from build123d import *

# Parameters (mm, degrees)
F2_DEPTH = 1.3
F4_DEPTH = 1.7
F6_DEPTH = 12.5


# Not quite as in the source:
# - a feature of the source that left no trace in its solid (it failed there, or was rolled back) is left out


with BuildPart() as f2:
    # F1 (on Top) → F2 (new body)
    with BuildSketch(Plane.XY):
        with BuildLine():
            Line((-5.1537473182, 3.6727124144), (-5.7416372565, -3.0469003289))
            ThreePointArc((-5.7416372565, -3.0469003289), (0, -6.5), (5.7416372565, -3.0469003289))
            Line((5.7416372565, -3.0469003289), (5.1537473182, 3.6727124144))
            Line((5.1537473182, 3.6727124144), (3.4859795486, 4.7765922388))
            Line((3.4859795486, 4.7765922388), (2.7272692442, 2.9260899627))
            ThreePointArc((2.7272692442, 2.9260899627), (0, -4), (-2.7272692442, 2.9260899627))
            Line((-2.7272692442, 2.9260899627), (-3.4859795486, 4.7765922388))
            Line((-3.4859795486, 4.7765922388), (-5.1537473182, 3.6727124144))
        make_face()
    extrude(amount=F2_DEPTH)

    # F3 (on face) → F4 (join)
    with BuildSketch(Plane.XY.offset(1.3)):
        with BuildLine():
            Line((-4.6721311475, -3.2651478589), (-5.3278688525, -3.723414225))
            ThreePointArc((-5.3278688525, -3.723414225), (0, -6.5), (5.3278688525, -3.723414225))
            Line((5.3278688525, -3.723414225), (4.6721311475, -3.2651478589))
            ThreePointArc((4.6721311475, -3.2651478589), (0, -5.7), (-4.6721311475, -3.2651478589))
        make_face()
    extrude(amount=F4_DEPTH)

    # F5 (on Right) → F6 (cut, symmetric)
    with BuildSketch(Plane.YZ):
        Polygon((6.7765922388, 1.3), (2.9260899627, 1.3), (6.7765922388, -0.9230885256), align=None)
    extrude(amount=F6_DEPTH, both=True, mode=Mode.SUBTRACT)


solid = f2.part
Geometry check sheet. Reference: the model listing, model coordinates, mm. A direction names the side the tool comes from. Round coordinates to 2 decimals unless told otherwise and drop trailing zeros. Loops run counter-clockwise (first coordinate to the right, second up) from the corner with the lowest first, then second, coordinate; pieces in that order, holes last.
Item 1: Access from +Z, -Z, +X, -X, +Y, -Y to the whole of each face (thin tool, end or side, straight path). Record for faces 1 (the flat face through (-0.1, -4.2, 1.3)), 2 (the flat face through (0, -6, 3)), 3 (the flat face through (3.03, 3.66, 0.5)).
Item 2: Cross-section at A-A on x = 0. Record the boundary of the cut face in (y, z), then the cut area to 3 significant figures.
Item 3: Gauge pin test, flat ends, axial feed: pin 1 (6.5 mm diameter, centred on x = 0, y = 0, fed in from +Z); pin 2 (3 mm diameter, centred on x = -2.5, y = -0.5, fed in from +Z); pin 3 (1.5 mm diameter, centred on x = 0.5, z = 1.5, fed in from +Y). Record the tip position at first contact, or that the pin passes through.
Item 4: Cross-section at C-C on z = 1.1. Record the boundary of the cut face in (x, y).
Item 5: Cross-section at D-D on x = 1.5. Record the boundary of the cut face in (y, z), then the cut area to 3 significant figures.
Item 6: Cross-section at B-B on y = 0. Record the boundary of the cut face in (x, z).
Item 7: Thickness scan on line 1 (Y direction, x = 0, z = 1.05); line 2 (Z direction, x = 3, y = -4.5); line 3 (X direction, y = 0, z = 0.5). Record the ranges inside material, lowest first.
Answer sheet:
1. face 1: +Z, +Y
1. face 2: +Z, +X, -X, +Y, -Y
1. face 3: +Z, -Z, +Y
2. outline: (-6.5, 0) - (-4, 0) - (-4, 1.3) - (-5.7, 1.3) - (-5.7, 3) - (-6.5, 3) - close
2. area: 4.61 mm2
3. pin 1: passes through
3. pin 2: stops at z = 1.3
3. pin 3: stops at y = -3.81
4. outline: (-5.74, -3.05) arc R6.5 ccw to (5.74, -3.05) - (5.19, 3.27) - (2.87, 3.27) - (2.73, 2.93) arc R4 cw (long way) to (-2.73, 2.93) - (-2.87, 3.27) - (-5.19, 3.27) - close
5. outline: (-6.32, 0) - (-3.71, 0) - (-3.71, 1.3) - (-5.5, 1.3) - (-5.5, 3) - (-6.32, 3) - close
5. area: 4.80 mm2
6. outline: (-5.48, 0) - (-4, 0) - (-4, 1.3) - (-5.48, 1.3) - close; (4, 0) - (5.48, 0) - (5.48, 1.3) - (4, 1.3) - close
7. line 1: y = -6.5 to -4
7. line 2: z = 0 to 1.3
7. line 3: x = -5.48 to -4, 4 to 5.48
